The model under review builds one solid part; all positions refer to its coordinate system, in mm. Round coordinates to 2 decimals unless told otherwise and drop trailing zeros. Write each loop counter-clockwise with the first axis right and the second up, starting at its lowest first coordinate (ties: lowest second). Pieces come first, ordered by that corner, then holes. Notation, with made-up numbers: (72.5, -12) -> (111.5, -12) arc R30 cw to (111.5, 20) -> close; hole circle Ø5 at (-20.75, -11.75). An arc over 180 degrees is marked (long way). Answer in a Markdown table with one row per item. Add a question column.
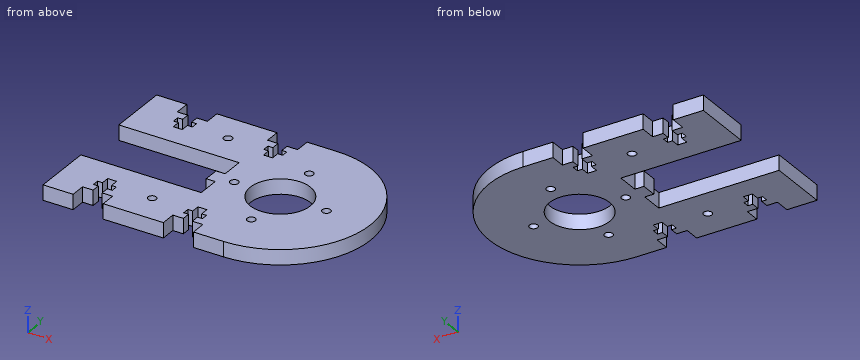
```python
from build123d import *

# Parameters (mm, degrees)
BOSS_EXTRUDE1_DEPTH  = 6.35
SKETCH2_W            = 50.8
SKETCH2_H            = 25.4
CUT_EXTRUDE1_DEPTH   = 86.430512699
CUT_EXTRUDE2_DEPTH   = 6.35
LPATTERN1_COUNT      = 2
LPATTERN1_PITCH      = 38.1
SKETCH4_R            = 1.7526
CUT_EXTRUDE5_DEPTH   = 86.430512699
SKETCH6_W            = 6.35
SKETCH6_H            = 6.604
BOSS_EXTRUDE2_DEPTH  = 3.81
MIRROR4_COPY_1_DEPTH = 6.35
SKETCH5_R            = 12.7
CUT_EXTRUDE4_DEPTH   = 86.430512699
SKETCH7_R            = 1.7526
CUT_EXTRUDE6_DEPTH   = 86.430512699
CIRPATTERN1_COUNT    = 4


with BuildPart() as part:
    # Sketch1 → Boss-Extrude1 (new body)
    with BuildSketch(Plane.XY):
        with BuildLine():
            Line((-38.1, -38.1), (38.1, -38.1))
            ThreePointArc((38.1, -38.1), (76.2, 0), (38.1, 38.1))
            Line((38.1, 38.1), (-38.1, 38.1))
            Line((-38.1, 38.1), (-38.1, -38.1))
        make_face()
    extrude(amount=BOSS_EXTRUDE1_DEPTH)

    # Sketch2 → Cut-Extrude1 (cut, through all)
    with BuildSketch(Plane.XY.offset(6.35)):
        with Locations((-12.7, 0)):
            Rectangle(SKETCH2_W, SKETCH2_H)
    extrude(amount=-CUT_EXTRUDE1_DEPTH, mode=Mode.SUBTRACT)

    # Sketch3 → Cut-Extrude2 (cut)
    with BuildSketch(Plane.XY.offset(6.35)):
        Polygon((-25.4, -38.1), (-12.7, -38.1), (-12.7, -31.75), (-17.15135, -31.75), (-17.15135, -28.2495625), (-15.08125, -28.2495625), (-15.08125, -25.4714375), (-17.15135, -25.4714375), (-17.15135, -21.971), (-20.94865, -21.971), (-20.94865, -25.4714375), (-23.01875, -25.4714375), (-23.01875, -28.2495625), (-20.94865, -28.2495625), (-20.94865, -31.75), (-25.4, -31.75), align=None)
    cut_extrude2 = extrude(amount=-CUT_EXTRUDE2_DEPTH, mode=Mode.SUBTRACT)

    # LPattern1: Cut-Extrude2 ×2
    with Locations(*[(i * LPATTERN1_PITCH, 0, 0) for i in range(1, LPATTERN1_COUNT)]):
        add(cut_extrude2, mode=Mode.SUBTRACT)

    # Sketch4 → Cut-Extrude5 (cut, through all)
    with BuildSketch(Plane.XY.offset(6.35)):
        with Locations((0, -25.4)):
            Circle(SKETCH4_R)
    cut_extrude5 = extrude(amount=-CUT_EXTRUDE5_DEPTH, mode=Mode.SUBTRACT)

    # Sketch6 → Boss-Extrude2 (add)
    with BuildSketch(Plane.ZY.offset(-12.7)):
        with Locations((3.175, 0)):
            Rectangle(SKETCH6_W, SKETCH6_H)
    extrude(amount=BOSS_EXTRUDE2_DEPTH)

    # Mirror3: Cut-Extrude5 across plane
    add(cut_extrude5.mirror(Plane.ZX), mode=Mode.SUBTRACT)

    # Mirror4: Cut-Extrude2 across plane
    add(cut_extrude2.mirror(Plane.ZX), mode=Mode.SUBTRACT)

    # Mirror4 copy 1 sketch → Mirror4 copy 1 (cut)
    with BuildSketch(Plane(origin=(38.1, 0, 6.35), x_dir=(1, 0, 0), z_dir=(0, 0, 1))):
        Polygon((-25.4, 38.1), (-12.7, 38.1), (-12.7, 31.75), (-17.15135, 31.75), (-17.15135, 28.2495625), (-15.08125, 28.2495625), (-15.08125, 25.4714375), (-17.15135, 25.4714375), (-17.15135, 21.971), (-20.94865, 21.971), (-20.94865, 25.4714375), (-23.01875, 25.4714375), (-23.01875, 28.2495625), (-20.94865, 28.2495625), (-20.94865, 31.75), (-25.4, 31.75), align=None)
    extrude(amount=-MIRROR4_COPY_1_DEPTH, mode=Mode.SUBTRACT)

    # Sketch5 → Cut-Extrude4 (cut, through all)
    with BuildSketch(Plane.XY.offset(6.35)):
        with Locations((38.1, 0)):
            Circle(SKETCH5_R)
    extrude(amount=-CUT_EXTRUDE4_DEPTH, mode=Mode.SUBTRACT)

    # Sketch7 → Cut-Extrude6 (cut, through all)
    with BuildSketch(Plane.XY.offset(6.35)):
        with Locations((38.1, 19.4437)):
            Circle(SKETCH7_R)
    cut_extrude6 = extrude(amount=-CUT_EXTRUDE6_DEPTH, mode=Mode.SUBTRACT)

    # CirPattern1: Cut-Extrude6 ×4 about axis
    cirpattern1_axis = Axis((38.1, 0, 0), (0, 0, 1))
    for i in range(1, CIRPATTERN1_COUNT):
        add(cut_extrude6.rotate(cirpattern1_axis, i * 360 / CIRPATTERN1_COUNT), mode=Mode.SUBTRACT)


solid = part.part
```
1. Insertion check: pin 1 Ø5.5 at (x, y) = (57.54, 0) entering from -Z; pin 2 Ø1.1 at (x, z) = (-20, 3.5) entering from +Y; pin 3 Ø1.8 at (y, z) = (-24, 2.5) entering from +X; pin 4 Ø3 at (x, z) = (-23.5, 3.5) entering from -Y. Each pin has a flat end and moves straight along its axis. Give the tip position at first contact, or say it passes through.
2. Add section B-B on y = 0. Write out the cut boundary in (x, z), plus the area to 3 significant figures.
3. Add section C-C on x = 43. Write out the cut boundary in (y, z).
4. Add section A-A on x = 0. Write out the cut boundary in (y, z).
5. For L1, parallel to X at y = -26, z = 1.5; L2, parallel to X at y = 27.5, z = 4.75; L3, parallel to Y at x = -3.5, z = 1.25, list the stretches that pass through material, from the lowest coordinate up.
6. Add section D-D on x = 31. Write out the cut boundary in (y, z).
Filled in:
| question | item | result |
|---|---|---|
| 1 | pin 1 | z = 0 |
| 1 | pin 2 | y = 21.97 |
| 1 | pin 3 | x = 68.4 |
| 1 | pin 4 | y = -31.75 |
| 2 | outline | (8.89, 0) -> (16.9, 0) -> (16.9, 6.35) -> (8.89, 6.35) -> close; (20.41, 0) -> (25.4, 0) -> (25.4, 6.35) -> (20.41, 6.35) -> close; (50.8, 0) -> (55.79, 0) -> (55.79, 6.35) -> (50.8, 6.35) -> close; (59.3, 0) -> (76.2, 0) -> (76.2, 6.35) -> (59.3, 6.35) -> close |
| 2 | area | 222 mm² |
| 3 | outline | (-37.78, 0) -> (-11.72, 0) -> (-11.72, 6.35) -> (-37.78, 6.35) -> close; (11.72, 0) -> (37.78, 0) -> (37.78, 6.35) -> (11.72, 6.35) -> close |
| 4 | outline | (-38.1, 0) -> (-27.15, 0) -> (-27.15, 6.35) -> (-38.1, 6.35) -> close; (-23.65, 0) -> (-12.7, 0) -> (-12.7, 6.35) -> (-23.65, 6.35) -> close; (12.7, 0) -> (23.65, 0) -> (23.65, 6.35) -> (12.7, 6.35) -> close; (27.15, 0) -> (38.1, 0) -> (38.1, 6.35) -> (27.15, 6.35) -> close |
| 5 | L1 | -38.1 to -23.02, -15.08 to -1.65, 1.65 to 15.08, 23.02 to 65.95 |
| 5 | L2 | -38.1 to -23.02, -15.08 to 15.08, 23.02 to 64.47 |
| 5 | L3 | -38.1 to -12.7, 12.7 to 38.1 |
| 6 | outline | (-38.1, 0) -> (-10.53, 0) -> (-10.53, 6.35) -> (-38.1, 6.35) -> close; (10.53, 0) -> (38.1, 0) -> (38.1, 6.35) -> (10.53, 6.35) -> close |
